Geometry: final body of the model. Coordinates: model frame, mm. A direction names the side the tool comes from. Round coordinates to 2 decimals unless told otherwise and drop trailing zeros. Loops run counter-clockwise (first coordinate to the right, second up) from the corner with the lowest first, then second, coordinate; pieces in that order, holes last. Notation, with made-up numbers: (-5, 63) - (19, 63) arc R35 ccw to (19, 100) - close; hole circle Ø10 at (2.25, 76.25). An arc over 180 degrees is marked (long way). Answer in a Markdown table with one row per item. Add a question column.
Autodesk Inventor part; units mm, degrees
ref_plane "YZ Plane" through (0, 0, 0) normal (1, 0, 0) x (0, 1, 0)
ref_plane "XZ Plane" through (0, 0, 0) normal (0, 1, 0) x (-1, 0, 0)
ref_plane "XY Plane" through (0, 0, 0) normal (0, 0, 1) x (1, 0, 0)
sketch "Эскиз1" plane through (0, 0, 0) normal (0, 0, 1) x (1, 0, 0)
  line L0 (0, 0) -> (15, 0)
  line L1 (15, 0) -> (15, 30)
  line L2 (15, 30) -> (20, 30)
  line L3 (20, 30) -> (20, 310)
  line L4 (20, 310) -> (45, 310)
  line L5 (45, 310) -> (45, 320)
  line L6 (45, 320) -> (55, 320)
  line L7 (55, 320) -> (55, 340)
  line L8 (55, 340) -> (60, 340)
  line L9 (60, 340) -> (60, 347)
  line L10 (52, 355) -> (0, 355)
  arc A0 (60, 347) -> (52, 355) centre (52, 347) ccw
  line L11 (15, 0) -> (10, 0)
  line L12 (10, 0) -> (10, 35)
  line L13 (10, 35) -> (15, 35)
  line L14 (15, 35) -> (15, 315)
  line L15 (15, 315) -> (40, 315)
  line L16 (40, 315) -> (40, 325)
  line L17 (40, 325) -> (50, 325)
  line L18 (50, 325) -> (50, 343.5)
  line L19 (50, 343.5) -> (55, 343.5)
  line L20 (55, 343.5) -> (55, 346.5)
  line L21 (51, 350.5) -> (0, 350.5)
  arc A1 (55, 346.5) -> (51, 350.5) centre (51, 346.5) ccw
  line L22 (0, 355) -> (0, 350.5)
  point P0 (60, 355)
  dimension "d0" = 15
  dimension "d1" = 30
  dimension "d2" = 5
  dimension "d3" = 280
  dimension "d4" = 25
  dimension "d5" = 10
  dimension "d6" = 10
  dimension "d7" = 20
  dimension "d8" = 5
  dimension "d9" = 15
  dimension "d10" = 8
  dimension "d11" = 5
  dimension "d12" = 35
  dimension "d13" = 25
  dimension "d14" = 10
  dimension "d15" = 10
  dimension "d16" = 18.5
  dimension "d17" = 4
  dimension "d18" = 3
revolve "Вращение1" add sketch "Эскиз1" angle 360 about axis through (0, 355, 0) along (0, -1, 0)
sketch "Эскиз2" plane through (0, 0, 0) normal (1, 0, 0) x (0, 1, 0)
  line L0 (340, 55) -> (340, -55)
  line L1 (320, 55) -> (320, -55)
  circle A0 centre (330, 0) radius 2.5
  point P0 (0, 0)
  dimension "d20" = 5
extrude "Выдавливание1" cut sketch "Эскиз2" against normal through all both and the other way through all
pattern_circular "Круговой массив1" count 4 over 360 about axis through (0, 330, 0) along (0, -1, 0) of "Выдавливание1"
thread "Резьба1"
chamfer "Фаска1" distance 2 angle 45 1 edges at (-15, 0, 0)
properties part number "Сапун" material "Чугун, серый"
1) Pull-direction query (Y, two-part tool) for faces 1 (the cylindrical face through (-14.985, 16.196, -0.66)), 2 (the flat face through (7, 0, -8)), 3 (the flat face through (12, 343.5, -49)); classes: pulls with the +Y half, pulls with the -Y half, needs draft (parallel to the pull), parting line crosses it, or undercut.
2) Reachability of faces 4 (the cylindrical face through (-11.923, 345.021, 53.692)), 5 (the flat face through (9, 310, -19)), 6 (the cylindrical face through (-59.94, 343.55, -2.64)) from +Z, -Z, +X, -X, +Y, -Y: full face, straight path, thin tool, end or side. Return the list, or none.
3) Section A-A, the plane y = 305.5. Return the cut outline in (x, z), and give its area (3 significant figures).
4) Material intervals for line 1 along Y through (x, z) = (-1.5, -37); line 2 along Z through (x, y) = (0, 174.5); line 3 along Y through (x, z) = (0, 52), sorted ascending. Write a range as from..to.
5) Contact query for flat-ended pins moving along their axis: pin 1 Ø6 at (y, z) = (330, 0) entering from +X; pin 2 Ø3 at (x, y) = (17.5, 103.5) entering from -Z; pin 3 Ø2 at (x, y) = (16.5, 181.5) entering from +Z. Output: stop coordinate, or through.
Evaluation:
| question | item | result |
|---|---|---|
| 1 | face 1 | needs draft |
| 1 | face 2 | pulls with the -Y half |
| 1 | face 3 | undercut |
| 2 | face 4 | none |
| 2 | face 5 | -Y |
| 2 | face 6 | +Y, -Y |
| 3 | outline | circle Ø40 at (0, 0); hole circle Ø30 at (0, 0) |
| 3 | area | 550 mm² |
| 4 | line 1 | y = 310..315, 350.5..355 |
| 4 | line 2 | z = -20..-15, 15..20 |
| 4 | line 3 | y = 320..327.5, 332.5..343.5, 350.37..355 |
| 5 | pin 1 | stops at x = 55 |
| 5 | pin 2 | stops at z = -12 |
| 5 | pin 3 | stops at z = 12.64 |
